Source: CAD feature listing. Evaluate the final solid. Frame: model axes, mm. A direction names the side the tool comes from. Give positions to 0.01 mm unless a question says otherwise; leave off trailing zeros. Order: outer loops, then holes, each group sorted by start corner. A loop starts at its lowest first (then second) coordinate and runs counter-clockwise, first axis right, second up. Notation, with made-up numbers: M -27.5,-33 L 16.5,-33 A15 ccw 16.5,-14 Z; hole C 64,89 d9. An arc over 180 degrees is marked long. Answer as a JSON object with one key per item and string values. Group by question number.
1. Pin query (flat end, axial travel): P1, Ø16, axis at y = -37.5, z = -869.5, coming from the +X side; P2, Ø13.5, axis at y = -3, z = -547.5, coming from the -X side; P3, Ø12, axis at y = 32, z = -14, coming from the +X side. Return the tip coordinate at first contact, or that it passes through.
2. Section query B-B (x = 245.5). Output: boundary loops of the cut face in (y, z).
3. Material intervals for L1, parallel to Y at x = 260, z = -264; L2, parallel to Z at x = 196.5, y = 29.5; L3, parallel to X at y = -6, z = -95, sorted ascending. Write a range as [from, to].
4. Section query A-A (z = -270). Output: boundary loops of the cut face in (x, y), plus the area to 3 significant figures.
5. Set-up query: faces 5 (the flat face through (199, -1, -860)), 6 (the flat face through (200.519, -34, -15)), 7 (the flat face through (202.42, 32, -15)). Return all of +Z, -Z, +X, -X, +Y, -Y with unobstructed straight access to the full face (end or side cutting, diameter ignored); none if empty.
6. Pull-direction query (Z, two-part tool) for faces 1 (the flat face through (223, 1, 0)), 2 (the flat face through (199, -1, -30)), 3 (the flat face through (224, 20.22, -443)), 4 (the flat face through (217.42, -2, -451)); classes: +Z half, -Z half, draft (parallel to the pull), parting line (faces both ways), or undercut.
from build123d import *

# Parameters (mm, degrees)
BOSS_EXTRUDE1_DEPTH = 890
SKETCH2_W           = 830
SKETCH2_H           = 88.44
CUT_EXTRUDE1_DEPTH  = 30


with BuildPart() as part:
    # Sketch1 → Boss-Extrude1 (new body)
    with BuildSketch(Plane.XY):
        with BuildLine():
            Line((187.42, 44.22), (187.42, -44.22))
            Line((187.42, -44.22), (200.51881238, -44.22))
            Line((200.51881238, -44.22), (200.51881238, -24.22))
            Line((200.51881238, -24.22), (280.51881238, -24.22))
            Line((280.51881238, -24.22), (280.51881238, 3.445359838))
            ThreePointArc((280.51881238, 3.445359838), (250.085390083, 1.968696909), (225.68736431, 20.22))
            Line((225.68736431, 20.22), (202.42, 20.22))
            Line((202.42, 20.22), (202.42, 44.22))
            Line((202.42, 44.22), (187.42, 44.22))
        make_face()
    extrude(amount=-BOSS_EXTRUDE1_DEPTH)

    # Sketch2 → Cut-Extrude1 (cut)
    with BuildSketch(Plane.ZY.offset(-187.42)):
        with Locations((-445, 0)):
            Rectangle(SKETCH2_W, SKETCH2_H)
    extrude(amount=-CUT_EXTRUDE1_DEPTH, mode=Mode.SUBTRACT)


solid = part.part
Answer sheet:
{
 "1": {"P1": "x = 200.52", "P2": "x = 217.42", "P3": "x = 202.42"},
 "2": {"outline": "M -24.22,-890 L 3.65,-890 L 3.65,0 L -24.22,0 Z"},
 "3": {"L1": "[-24.22, 0.12]", "L2": "[-890, -860], [-30, 0]", "L3": "[217.42, 280.52]"},
 "4": {"outline": "M 217.42,-24.22 L 280.52,-24.22 L 280.52,3.45 A45 cw 225.69,20.22 L 217.42,20.22 Z", "area": "1,940 mm^2"},
 "5": {"face 5": "-X, +Y, -Y", "face 6": "+Z, -Z, +X, -Y", "face 7": "+Z, -Z, +X, +Y"},
 "6": {"face 1": "+Z half", "face 2": "undercut", "face 3": "draft", "face 4": "undercut"}
}
